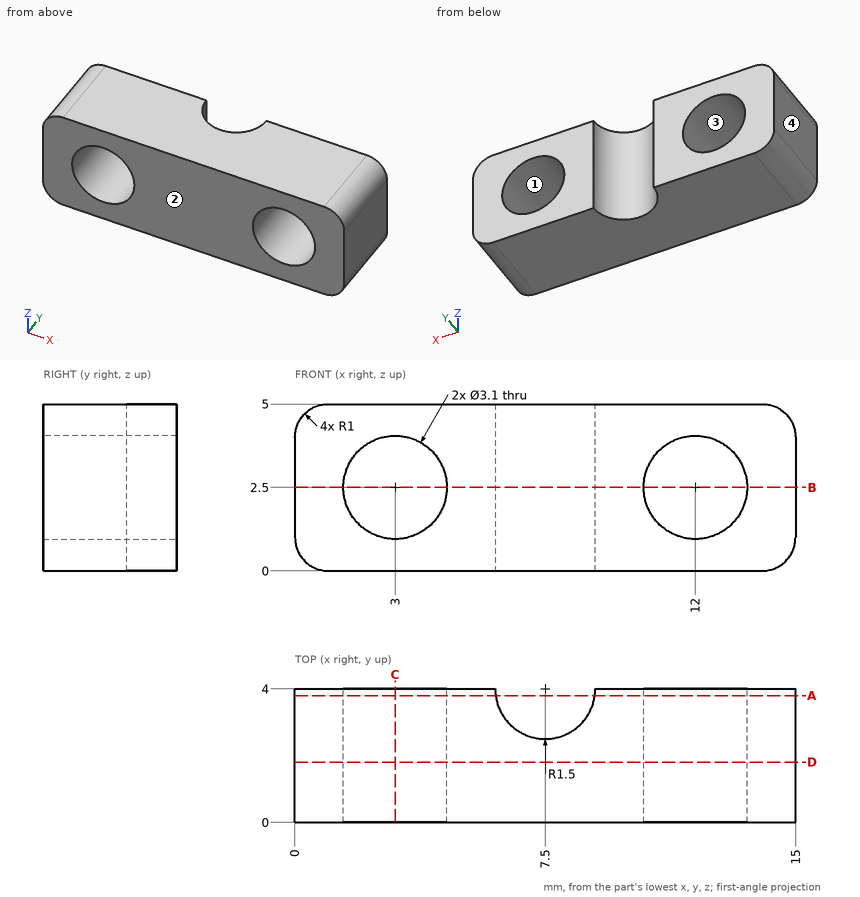
Job drawing, mm, ordinate dimensions from the low corner. One solid piece. Coordinates: 2 decimals unless noted, no trailing zeros. Order: outer loops, then holes, each group sorted by start corner. A loop starts at its lowest first (then second) coordinate and runs counter-clockwise, first axis right, second up. Notation, with made-up numbers: M 63,-39 L 86,-39 A37 cw 86,-3 Z; hole C 46.25,32 d6. An arc over 180 degrees is marked long. One line per question, with ' | ' between items.
Q1. Slice it at B-B (z = 2.5). Give the cut face in (x, y), and give its area (3 significant figures).
A:
outline: M 0,0 L 1.45,0 L 1.45,4 L 0,4 Z; M 4.55,0 L 10.45,0 L 10.45,4 L 9,4 A1.5 cw 6,4 L 4.55,4 Z; M 13.55,0 L 15,0 L 15,4 L 13.55,4 Z | area: 31.7 mm^2
Q2. Slice it at D-D (y = 1.8). Give the cut face in (x, z).
A:
outline: M 0,1 A1 ccw 1,0 L 14,0 A1 ccw 15,1 L 15,4 A1 ccw 14,5 L 1,5 A1 ccw 0,4 Z; hole C 3,2.5 d3.1; hole C 12,2.5 d3.1
Q3. Drill centre lines: line 1 (X direction, y = 2.2, z = 2.5); line 2 (X direction, y = 3.1, z = 1.5); line 3 (X direction, y = 3.5, z = 1.2). Where is each one in solid material? Low to high.
A:
line 1: x = 0 to 1.45, 4.55 to 10.45, 13.55 to 15 | line 2: x = 0 to 1.82, 4.18 to 6.3, 8.7 to 10.82, 13.18 to 15 | line 3: x = 0 to 2.16, 3.84 to 6.09, 8.91 to 11.16, 12.84 to 15
Q4. Pin check, flat tip, straight feed: P1, Ø2.5, axis at x = 3, z = 2.5, coming from the -Y side. Stop position of the tip, or through.
A:
P1: passes through
Q5. Slice it at C-C (x = 3). Give the cut face in (y, z), and give its area (3 significant figures).
A:
outline: M 0,0 L 4,0 L 4,0.95 L 0,0.95 Z; M 0,4.05 L 4,4.05 L 4,5 L 0,5 Z | area: 7.60 mm^2
Q6. Slice it at A-A (y = 3.8). Give the cut face in (x, z), and give its area (3 significant figures).
A:
outline: M 0,1 A1 ccw 1,0 L 6.01,0 L 6.01,5 L 1,5 A1 ccw 0,4 Z; M 8.99,0 L 14,0 A1 ccw 15,1 L 15,4 A1 ccw 14,5 L 8.99,5 Z; hole C 3,2.5 d3.1; hole C 12,2.5 d3.1 | area: 44.2 mm^2
Q7. Two-plate mould, pull along X, no slides. Class the marked faces 1, 2, 3 and 4: +X half, -X half, draft (parallel to the pull), parting line (faces both ways), or undercut.
A:
face 1: undercut | face 2: draft | face 3: undercut | face 4: -X half
